Read the model definition and answer for the solid it produces. Units are mm, in the model's axes. A direction names the side the tool comes from. Coordinates: 2 decimals unless noted, no trailing zeros. Write each loop counter-clockwise with the first axis right and the second up, starting at its lowest first coordinate (ties: lowest second). Pieces come first, ordered by that corner, then holes. Notation, with made-up numbers: (42, 62.5) -> (96, 62.5) arc R14 cw to (96, 83.5) -> close; hole circle Ø1 at (-2.5, 37.25). An arc over 180 degrees is marked (long way). Return JSON: item names as keys, results as strings.
from build123d import *

# Parameters (mm, degrees)
F0_W     = 140
F0_H     = 80
F0_W_2   = 20
F0_H_2   = 30
F1_DEPTH = 2.5


with BuildPart() as f1:
    # F0 (on Front) → F1 (new body, symmetric)
    with BuildSketch(Plane.XZ):
        with Locations((-70, 40)):
            Rectangle(F0_W, F0_H)
        with Locations((-115, 40)):
            Rectangle(F0_W_2, F0_H_2, mode=Mode.SUBTRACT)
        with Locations((-25, 40)):
            Rectangle(F0_W_2, F0_H_2, mode=Mode.SUBTRACT)
        Polygon((-140, 80), (0, 80), (0, 130), (-69.061231, 180), (-140, 130), align=None)
        with Locations((-115, 110)):
            Rectangle(F0_W_2, F0_H_2, mode=Mode.SUBTRACT)
        with Locations((-25, 110)):
            Rectangle(F0_W_2, F0_H_2, mode=Mode.SUBTRACT)
    extrude(amount=F1_DEPTH, both=True)


solid = f1.part
1. The part is cut by section D-D (x = -99.5). Determine the outline of the cut face in (y, z), then the cut area to 3 significant figures.
Taken from the geometry:
{"outline": "(-2.5, 0) -> (2.5, 0) -> (2.5, 158.55) -> (-2.5, 158.55) -> close", "area": "793 mm2"}
2. The part is cut by section A-A (z = 100.5). Determine the outline of the cut face in (x, y), then the cut area to 3 significant figures.
Taken from the geometry:
{"outline": "(-140, -2.5) -> (-125, -2.5) -> (-125, 2.5) -> (-140, 2.5) -> close; (-105, -2.5) -> (-35, -2.5) -> (-35, 2.5) -> (-105, 2.5) -> close; (-15, -2.5) -> (0, -2.5) -> (0, 2.5) -> (-15, 2.5) -> close", "area": "500 mm2"}
3. The part is cut by section C-C (y = 1.2). Determine the outline of the cut face in (x, z).
Taken from the geometry:
{"outline": "(-140, 0) -> (0, 0) -> (0, 130) -> (-69.06, 180) -> (-140, 130) -> close; hole (-125, 25) -> (-105, 25) -> (-105, 55) -> (-125, 55) -> close; hole (-125, 95) -> (-105, 95) -> (-105, 125) -> (-125, 125) -> close; hole (-35, 25) -> (-15, 25) -> (-15, 55) -> (-35, 55) -> close; hole (-35, 95) -> (-15, 95) -> (-15, 125) -> (-35, 125) -> close"}
4. A tool of negligible diameter and unlimited length cuts with its end or side. For faces 1 (the face through (-71, -2.5, 71)), 2 (the face through (-115, 0, 125)), from which of +Z, -Z, +X, -X, +Y, -Y can it reach the whole face along a straight path? Write none if from no direction.
Taken from the geometry:
{"face 1": "+Z, -Z, +X, -X, -Y", "face 2": "+Y, -Y"}
5. Consider L1, parallel to X at y = 0.1, z = 96.5; L2, parallel to Z at x = -109, y = -2.1; L3, parallel to Z at x = -106, y = -1.9. Determine where each line is inside the solid, lowest interval first.
Taken from the geometry:
{"L1": "x = -140 to -125, -105 to -35, -15 to 0", "L2": "z = 0 to 25, 55 to 95, 125 to 151.85", "L3": "z = 0 to 25, 55 to 95, 125 to 153.96"}
6. For a pull along X with two mould halves and no side action, classify faces 3 (the face through (-71, 0, 0)), 4 (the face through (-25, 0, 55)), 5 (the face through (-34.05, -0.04, 154.65)) as +X half, -X half, draft (parallel to the pull), parting line (faces both ways), or undercut.
Taken from the geometry:
{"face 3": "draft", "face 4": "undercut", "face 5": "+X half"}
7. Flat-ended cylindrical pins translate along their axes: pin 1 Ø1.5 at (x, y) = (-110.5, 0.5) entering from +Z; pin 2 Ø2.5 at (x, y) = (-27, 1) entering from +Z; pin 3 Ø1.5 at (x, y) = (-26.5, -0.5) entering from +Z. Find the tip coordinate at first contact, or state that the pin passes through.
Taken from the geometry:
{"pin 1": "stops at z = 151.32", "pin 2": "stops at z = 150.45", "pin 3": "stops at z = 149.73"}
8. The part is cut by section B-B (x = -20.5). Determine the outline of the cut face in (y, z).
Taken from the geometry:
{"outline": "(-2.5, 0) -> (2.5, 0) -> (2.5, 25) -> (-2.5, 25) -> close; (-2.5, 55) -> (2.5, 55) -> (2.5, 95) -> (-2.5, 95) -> close; (-2.5, 125) -> (2.5, 125) -> (2.5, 144.84) -> (-2.5, 144.84) -> close"}
